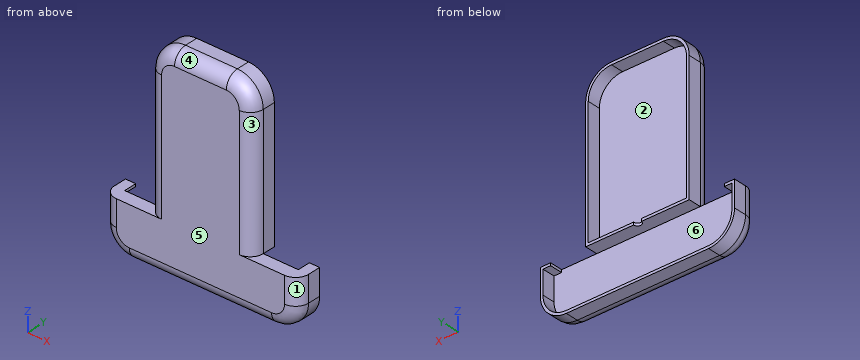
```python
from build123d import *

# Parameters (mm, degrees)
BOSS_EXTRUDE1_DEPTH  = 25.4
FILLET1_R            = 12.7
FILLET3_R            = 25.4
FILLET4_R            = 25.4
FILLET5_R            = 25.4
SHELL1_T             = -2.54
EXTRUDE_THIN1_REACH  = 252.592
SKETCH2_W            = 2.54
SKETCH2_H            = 198.12
EXTRUDE_THIN4_REACH  = 252.592
SKETCH3_W            = 47.014483258
SKETCH3_H            = 2.54
SKETCH3_W_2          = 47.014483257
EXTRUDE_THIN5_REACH  = 252.592
SKETCH5_W            = 47.014483258
SKETCH5_H            = 2.54
SKETCH5_W_2          = 47.014483257
EXTRUDE_THIN10_START = 10.16
EXTRUDE_THIN10_DEPTH = 2.54
EXTRUDE_THIN11_START = 10.16
EXTRUDE_THIN11_DEPTH = 2.54
CUT_EXTRUDE2_REACH   = 214.64
SKETCH11_W           = 34.417
SKETCH11_H           = 12.7
CUT_EXTRUDE3_REACH   = 253.556
SKETCH12_W           = 2.54
SKETCH12_H           = 12.7
CUT_EXTRUDE4_REACH   = 253.556
SKETCH13_W           = 2.54
SKETCH13_H           = 12.7
SKETCH14_W           = 96.568966515
SKETCH14_H           = 2.54
EXTRUDE_THIN13_DEPTH = 12.7
CUT_EXTRUDE6_REACH   = 212.827


with BuildPart() as part:
    # Sketch1 → Boss-Extrude1 (new body)
    with BuildSketch(Plane(origin=(0, 0, 0), x_dir=(1, 0, 0), z_dir=(0, 1, 0))):
        Polygon((0, 0), (0, 152.4), (-44.45, 152.4), (-44.45, 203.2), (146.098966515, 203.2), (146.098966515, 152.4), (101.648966515, 152.4), (101.648966515, 0), align=None)
    extrude(amount=BOSS_EXTRUDE1_DEPTH)

    # Fillet1
    fillet1_edges = [part.edges().sort_by_distance(p)[0] for p in [
        (146.098966515, 0, -177.8),
        (101.648966515, 0, -76.2),
        (50.824483258, 0, 0),
        (0, 0, -76.2),
        (-44.45, 0, -177.8),
        (50.824483258, 0, -203.2),
    ]]
    fillet(fillet1_edges, radius=FILLET1_R)

    # Fillet3
    # the kernel refuses this fillet: 25.4 mm, written as the material it takes off along each edge
    with BuildSketch(Plane(origin=(76.248966515, 0, -25.4), x_dir=(1, 0, 0), z_dir=(0, 0, -1))) as fillet3_piece_1:
        with BuildLine():
            CenterArc((12.7, -12.7), 12.7, 0, 90)
            Line((25.4, -12.7), (25.4, 0))
            Line((25.4, 0), (12.7, 0))
        make_face()
    revolve(axis=Axis((76.248966515, 0, -25.4), (0, -1, 0)), revolution_arc=90, mode=Mode.SUBTRACT)
    with BuildSketch(Plane(origin=(101.648966515, 0, 0), x_dir=(0, 0, -1), z_dir=(0, 1, 0))) as fillet3_piece_2:
        with BuildLine():
            CenterArc((FILLET3_R, FILLET3_R), FILLET3_R, 180, 90)
            Line((0, FILLET3_R), (0, 0))
            Line((0, 0), (FILLET3_R, 0))
        make_face()
    extrude(amount=88.9, mode=Mode.SUBTRACT)

    # Fillet4
    # the kernel refuses this fillet: 25.4 mm, written as the material it takes off along each edge
    with BuildSketch(Plane(origin=(25.4, 0, -25.4), x_dir=(0, 0, 1), z_dir=(1, 0, 0))) as fillet4_piece_1:
        with BuildLine():
            CenterArc((12.7, -12.7), 12.7, 0, 90)
            Line((25.4, -12.7), (25.4, 0))
            Line((25.4, 0), (12.7, 0))
        make_face()
    revolve(axis=Axis((25.4, 0, -25.4), (0, -1, 0)), revolution_arc=90, mode=Mode.SUBTRACT)
    with BuildSketch(Plane(origin=(0, 0, 0), x_dir=(0, 0, -1), z_dir=(0, 1, 0))) as fillet4_piece_2:
        with BuildLine():
            CenterArc((FILLET4_R, -FILLET4_R), FILLET4_R, 90, 90)
            Line((0, -FILLET4_R), (0, 0))
            Line((0, 0), (FILLET4_R, 0))
        make_face()
    extrude(amount=88.9, mode=Mode.SUBTRACT)

    # Fillet5
    # the kernel refuses this fillet: 25.4 mm, written as the material it takes off along each edge
    with BuildSketch(Plane(origin=(120.698966515, 0, -177.8), x_dir=(0, 0, -1), z_dir=(-1, 0, 0))) as fillet5_piece_1:
        with BuildLine():
            CenterArc((12.7, -12.7), 12.7, 0, 90)
            Line((25.4, -12.7), (25.4, 0))
            Line((25.4, 0), (12.7, 0))
        make_face()
    revolve(axis=Axis((120.698966515, 0, -177.8), (0, -1, 0)), revolution_arc=90, mode=Mode.SUBTRACT)
    with BuildSketch(Plane(origin=(-19.05, 0, -177.8), x_dir=(-1, 0, 0), z_dir=(0, 0, 1))) as fillet5_piece_2:
        with BuildLine():
            CenterArc((12.7, -12.7), 12.7, 0, 90)
            Line((25.4, -12.7), (25.4, 0))
            Line((25.4, 0), (12.7, 0))
        make_face()
    revolve(axis=Axis((-19.05, 0, -177.8), (0, -1, 0)), revolution_arc=90, mode=Mode.SUBTRACT)
    with BuildSketch(Plane(origin=(-44.45, 0, -203.2), x_dir=(0, 0, 1), z_dir=(0, 1, 0))) as fillet5_piece_3:
        with BuildLine():
            CenterArc((FILLET5_R, FILLET5_R), FILLET5_R, 180, 90)
            Line((0, FILLET5_R), (0, 0))
            Line((0, 0), (FILLET5_R, 0))
        make_face()
    extrude(amount=88.9, mode=Mode.SUBTRACT)
    with BuildSketch(Plane(origin=(146.098966515, 0, -203.2), x_dir=(0, 0, 1), z_dir=(0, 1, 0))) as fillet5_piece_4:
        with BuildLine():
            CenterArc((FILLET5_R, -FILLET5_R), FILLET5_R, 90, 90)
            Line((0, -FILLET5_R), (0, 0))
            Line((0, 0), (FILLET5_R, 0))
        make_face()
    extrude(amount=88.9, mode=Mode.SUBTRACT)

    # Shell1
    shell1_openings = [part.faces().sort_by_distance(p)[0] for p in [
        (50.824483258, 25.4, -115.579080846),
    ]]
    offset(amount=SHELL1_T, openings=shell1_openings, kind=Kind.INTERSECTION)

    # Sketch2 → Extrude-Thin1 (add, up to next)
    with BuildSketch(Plane(origin=(0, 12.7, 0), x_dir=(1, 0, 0), z_dir=(0, 1, 0)), mode=Mode.PRIVATE) as extrude_thin1_sk1:
        with Locations((50.824483258, 101.6)):
            Rectangle(SKETCH2_W, SKETCH2_H)
    extrude_thin1_tool1 = extrude(extrude_thin1_sk1.sketch, amount=-EXTRUDE_THIN1_REACH, mode=Mode.PRIVATE) - part.part
    add(extrude_thin1_tool1.solids().sort_by_distance((50.824483, 12.7, -101.6))[0])

    # Sketch3 → Extrude-Thin4 (add, up to next)
    with BuildSketch(Plane(origin=(0, 12.7, 0), x_dir=(1, 0, 0), z_dir=(0, 1, 0)), mode=Mode.PRIVATE) as extrude_thin4_sk1:
        with Locations((26.047241629, 66.04)):
            Rectangle(SKETCH3_W, SKETCH3_H)
    extrude_thin4_tool1 = extrude(extrude_thin4_sk1.sketch, amount=-EXTRUDE_THIN4_REACH, mode=Mode.PRIVATE) - part.part
    # Sketch3 → Extrude-Thin4 (add, up to next)
    with BuildSketch(Plane(origin=(0, 12.7, 0), x_dir=(1, 0, 0), z_dir=(0, 1, 0)), mode=Mode.PRIVATE) as extrude_thin4_sk2:
        with Locations((75.601724887, 66.04)):
            Rectangle(SKETCH3_W_2, SKETCH3_H)
    extrude_thin4_tool2 = extrude(extrude_thin4_sk2.sketch, amount=-EXTRUDE_THIN4_REACH, mode=Mode.PRIVATE) - part.part
    add(extrude_thin4_tool1.solids().sort_by_distance((26.047242, 12.7, -66.04))[0])
    add(extrude_thin4_tool2.solids().sort_by_distance((75.601725, 12.7, -66.04))[0])

    # Sketch5 → Extrude-Thin5 (add, up to next)
    with BuildSketch(Plane(origin=(0, 12.7, 0), x_dir=(1, 0, 0), z_dir=(0, 1, 0)), mode=Mode.PRIVATE) as extrude_thin5_sk1:
        with Locations((26.047241629, 143.51)):
            Rectangle(SKETCH5_W, SKETCH5_H)
    extrude_thin5_tool1 = extrude(extrude_thin5_sk1.sketch, amount=-EXTRUDE_THIN5_REACH, mode=Mode.PRIVATE) - part.part
    # Sketch5 → Extrude-Thin5 (add, up to next)
    with BuildSketch(Plane(origin=(0, 12.7, 0), x_dir=(1, 0, 0), z_dir=(0, 1, 0)), mode=Mode.PRIVATE) as extrude_thin5_sk2:
        with Locations((75.601724887, 143.51)):
            Rectangle(SKETCH5_W_2, SKETCH5_H)
    extrude_thin5_tool2 = extrude(extrude_thin5_sk2.sketch, amount=-EXTRUDE_THIN5_REACH, mode=Mode.PRIVATE) - part.part
    add(extrude_thin5_tool1.solids().sort_by_distance((26.047242, 12.7, -143.51))[0])
    add(extrude_thin5_tool2.solids().sort_by_distance((75.601725, 12.7, -143.51))[0])

    # Extrude-Thin10: read off the stored shape, not the designer's step
    # Extrude-Thin10 outline → Extrude-Thin10 (add)
    with BuildSketch(Plane(origin=(0, 0, 0), x_dir=(1, 0, 0), z_dir=(0, 1, 0)).offset(EXTRUDE_THIN10_START)):
        with BuildLine():
            ThreePointArc((2.54, 25.4), (9.235538982, 9.235538982), (25.4, 2.54))
            Line((25.4, 2.54), (52.094483258, 2.54))
            Line((52.094483258, 2.54), (52.094483258, 64.77))
            Line((52.094483258, 64.77), (99.108966515, 64.77))
            Line((99.108966515, 64.77), (99.108966515, 67.31))
            Line((99.108966515, 67.31), (52.094483258, 67.31))
            Line((52.094483258, 67.31), (52.094483258, 142.24))
            Line((52.094483258, 142.24), (99.108966515, 142.24))
            Line((99.108966515, 142.24), (99.108966515, 144.78))
            Line((99.108966515, 144.78), (52.094483258, 144.78))
            Line((52.094483258, 144.78), (52.094483258, 200.66))
            Line((52.094483258, 200.66), (-19.05, 200.66))
            ThreePointArc((-19.05, 200.66), (-35.214461018, 193.964461018), (-41.91, 177.8))
            Line((-41.91, 177.8), (-41.91, 154.94))
            Line((-41.91, 154.94), (2.54, 154.94))
            Line((2.54, 154.94), (2.54, 25.4))
        make_face()
    extrude(amount=EXTRUDE_THIN10_DEPTH)

    # Extrude-Thin11: read off the stored shape, not the designer's step
    # Extrude-Thin11 outline → Extrude-Thin11 (add)
    with BuildSketch(Plane(origin=(0, 0, 0), x_dir=(1, 0, 0), z_dir=(0, 1, 0)).offset(EXTRUDE_THIN11_START)):
        with BuildLine():
            ThreePointArc((2.54, 25.4), (9.235538982, 9.235538982), (25.4, 2.54))
            Line((25.4, 2.54), (76.248966515, 2.54))
            ThreePointArc((76.248966515, 2.54), (92.413427533, 9.235538982), (99.108966515, 25.4))
            Line((99.108966515, 25.4), (99.108966515, 154.94))
            Line((99.108966515, 154.94), (143.558966515, 154.94))
            Line((143.558966515, 154.94), (143.558966515, 177.8))
            ThreePointArc((143.558966515, 177.8), (136.863427533, 193.964461018), (120.698966515, 200.66))
            Line((120.698966515, 200.66), (-19.05, 200.66))
            ThreePointArc((-19.05, 200.66), (-35.214461018, 193.964461018), (-41.91, 177.8))
            Line((-41.91, 177.8), (-41.91, 154.94))
            Line((-41.91, 154.94), (2.54, 154.94))
            Line((2.54, 154.94), (2.54, 25.4))
        make_face()
    extrude(amount=EXTRUDE_THIN11_DEPTH)

    # Sketch11 → Cut-Extrude2 (cut, up to next)
    with BuildSketch(Plane.XY.offset(-152.4), mode=Mode.PRIVATE) as cut_extrude2_sk1:
        with Locations((-17.2085, 19.05)):
            Rectangle(SKETCH11_W, SKETCH11_H)
    cut_extrude2_tool1 = extrude(cut_extrude2_sk1.sketch, amount=-CUT_EXTRUDE2_REACH, mode=Mode.PRIVATE) & part.part
    # Sketch11 → Cut-Extrude2 (cut, up to next)
    with BuildSketch(Plane.XY.offset(-152.4), mode=Mode.PRIVATE) as cut_extrude2_sk2:
        with Locations((118.857466515, 19.05)):
            Rectangle(SKETCH11_W, SKETCH11_H)
    cut_extrude2_tool2 = extrude(cut_extrude2_sk2.sketch, amount=-CUT_EXTRUDE2_REACH, mode=Mode.PRIVATE) & part.part
    add(cut_extrude2_tool1.solids().sort_by_distance((-17.2085, 19.05, -152.4))[0], mode=Mode.SUBTRACT)
    add(cut_extrude2_tool2.solids().sort_by_distance((118.857467, 19.05, -152.4))[0], mode=Mode.SUBTRACT)

    # Sketch12 → Cut-Extrude3 (cut, up to next)
    with BuildSketch(Plane(origin=(101.648966515, 0, 0), x_dir=(0, 0, -1), z_dir=(1, 0, 0)), mode=Mode.PRIVATE) as cut_extrude3_sk1:
        with Locations((153.67, 19.05)):
            Rectangle(SKETCH12_W, SKETCH12_H)
    cut_extrude3_tool1 = extrude(cut_extrude3_sk1.sketch, amount=-CUT_EXTRUDE3_REACH, mode=Mode.PRIVATE) & part.part
    add(cut_extrude3_tool1.solids().sort_by_distance((101.648967, 19.05, -153.67))[0], mode=Mode.SUBTRACT)

    # Sketch13 → Cut-Extrude4 (cut, up to next)
    with BuildSketch(Plane.ZY, mode=Mode.PRIVATE) as cut_extrude4_sk1:
        with Locations((-153.67, 19.05)):
            Rectangle(SKETCH13_W, SKETCH13_H)
    cut_extrude4_tool1 = extrude(cut_extrude4_sk1.sketch, amount=-CUT_EXTRUDE4_REACH, mode=Mode.PRIVATE) & part.part
    add(cut_extrude4_tool1.solids().sort_by_distance((0, 19.05, -153.67))[0], mode=Mode.SUBTRACT)

    # Sketch14 → Extrude-Thin13 (add)
    with BuildSketch(Plane(origin=(0, 12.7, 0), x_dir=(1, 0, 0), z_dir=(0, 1, 0))):
        with Locations((50.824483258, 151.13)):
            Rectangle(SKETCH14_W, SKETCH14_H)
    extrude(amount=EXTRUDE_THIN13_DEPTH)

    # Sketch16 → Cut-Extrude6 (cut, up to next)
    with BuildSketch(Plane.XY.offset(-149.86), mode=Mode.PRIVATE) as cut_extrude6_sk1:
        with BuildLine():
            Line((47.014483258, 25.4), (54.634483258, 25.4))
            ThreePointArc((54.634483258, 25.4), (50.824483258, 21.59), (47.014483258, 25.4))
        make_face()
    cut_extrude6_tool1 = extrude(cut_extrude6_sk1.sketch, amount=-CUT_EXTRUDE6_REACH, mode=Mode.PRIVATE) & part.part
    add(cut_extrude6_tool1.solids().sort_by_distance((50.824483, 23.782986, -149.86))[0], mode=Mode.SUBTRACT)


solid = part.part
```
Verification items for the finished model (mm, model axes). Face numbers are marked on the shaded views. A direction names the side the tool comes from. Round coordinates to 2 decimals unless told otherwise and drop trailing zeros. Order: outer loops, then holes, each group sorted by start corner. A loop starts at its lowest first (then second) coordinate and runs counter-clockwise, first axis right, second up.
1) Depth check by flat-ended pin: pin 1 (2 mm diameter, centred on y = 11.5, z = -74.5, fed in from -X); pin 2 (5 mm diameter, centred on x = 102.5, z = -114, fed in from -Y); pin 3 (2.5 mm diameter, centred on y = 5, z = -94, fed in from +X). Enter the tip coordinate at first touch or a pass-through.
Geometry says:
pin 1: stops at x = 0
pin 2: stops at y = 6.44
pin 3: stops at x = 99.89
2) Cross-section at C-C, the plane z = -158.5. Record the cut outline in (x, y).
Geometry says:
outline: (-44.45, 12.7) arc R12.7 ccw to (-31.75, 0) - (133.4, 0) arc R12.7 ccw to (146.1, 12.7) - (146.1, 25.4) - (143.56, 25.4) - (143.56, 12.7) - (-41.91, 12.7) - (-41.91, 25.4) - (-44.45, 25.4) - close; hole (-41.59, 10.16) arc R10.16 ccw to (-31.75, 2.54) - (49.55, 2.54) - (49.55, 10.16) - close; hole (52.09, 2.54) - (133.4, 2.54) arc R10.16 ccw to (143.24, 10.16) - (52.09, 10.16) - close
3) Material ranges on line 1 (Z direction, x = 44.5, y = 20); line 2 (Y direction, x = 46.5, z = -121); line 3 (Z direction, x = 91, y = 5.75), recorded low to high.
Geometry says:
line 1: z = -203.2 to -200.66, -152.4 to -149.86, -2.54 to 0
line 2: y = 0 to 2.54, 10.16 to 12.7
line 3: z = -201.13 to -197.91, -144.78 to -142.24, -67.31 to -64.77, -11.73 to -7.33
4) Cross-section at A-A, the plane y = 16. Record the cut outline in (x, z).
Geometry says:
outline: (-44.45, -177.8) arc R25.4 ccw to (-19.05, -203.2) - (120.7, -203.2) arc R25.4 ccw to (146.1, -177.8) - (146.1, -152.4) - (136.07, -152.4) - (136.07, -154.94) - (143.56, -154.94) - (143.56, -177.8) arc R22.86 cw to (120.7, -200.66) - (-19.05, -200.66) arc R22.86 cw to (-41.91, -177.8) - (-41.91, -154.94) - (-34.42, -154.94) - (-34.42, -152.4) - (-44.45, -152.4) - close; (0, -152.4) - (101.65, -152.4) - (101.65, -25.4) arc R25.4 ccw to (76.25, 0) - (25.4, 0) arc R25.4 ccw to (0, -25.4) - close; hole (2.54, -149.86) - (99.11, -149.86) - (99.11, -25.4) arc R22.86 ccw to (76.25, -2.54) - (25.4, -2.54) arc R22.86 ccw to (2.54, -25.4) - close
5) Tool access check on the marked faces 1, 2 and 3. Record the directions out of +Z, -Z, +X, -X, +Y, -Y that give a thin tool (end or side, any length) a straight path to the whole face; none if there is none.
Geometry says:
face 1: +Z, -Z, +X, -Y
face 2: +Y
face 3: +Z, +X, -Y
6) Cross-section at D-D, the plane x = 118. Record the cut outline in (y, z).
Geometry says:
outline: (0, -190.5) arc R12.7 ccw to (12.7, -203.2) - (25.4, -203.2) - (25.4, -200.66) - (12.7, -200.66) - (12.7, -152.4) - (0, -152.4) - close; hole (2.54, -190.5) arc R10.16 ccw to (10.16, -200.34) - (10.16, -154.94) - (2.54, -154.94) - close
7) Cross-section at B-B, the plane x = 33.5. Record the cut outline in (y, z).
Geometry says:
outline: (0, -190.5) arc R12.7 ccw to (12.7, -203.2) - (25.4, -203.2) - (25.4, -200.66) - (12.7, -200.66) - (12.7, -152.4) - (25.4, -152.4) - (25.4, -149.86) - (12.7, -149.86) - (12.7, -2.54) - (25.4, -2.54) - (25.4, 0) - (12.7, 0) arc R12.7 ccw to (0, -12.7) - close; hole (2.54, -190.5) arc R10.16 ccw to (10.16, -200.34) - (10.16, -144.78) - (2.54, -144.78) - close; hole (2.54, -142.24) - (10.16, -142.24) - (10.16, -67.31) - (2.54, -67.31) - close; hole (2.54, -64.77) - (10.16, -64.77) - (10.16, -2.86) arc R10.16 ccw to (2.54, -12.7) - close
8) Draft check along Z on the marked faces 4, 5 and 6. Enter one of: +Z half, -Z half, draft (parallel to the pull), parting line (faces both ways), or undercut.
Geometry says:
face 4: +Z half
face 5: draft
face 6: undercut
